Part print with two shaded views. Sizes in mm from the minimum x, y, z corner. Give positions to 0.01 mm unless a question says otherwise; leave off trailing zeros. Loops run counter-clockwise (first coordinate to the right, second up) from the corner with the lowest first, then second, coordinate; pieces in that order, holes last. Notation, with made-up numbers: M 27.5,34.5 L 59.5,34.5 A19 cw 59.5,52.5 Z; hole C -27,60.25 d8. An arc over 180 degrees is marked long. Answer in a Markdown table with one row per item.
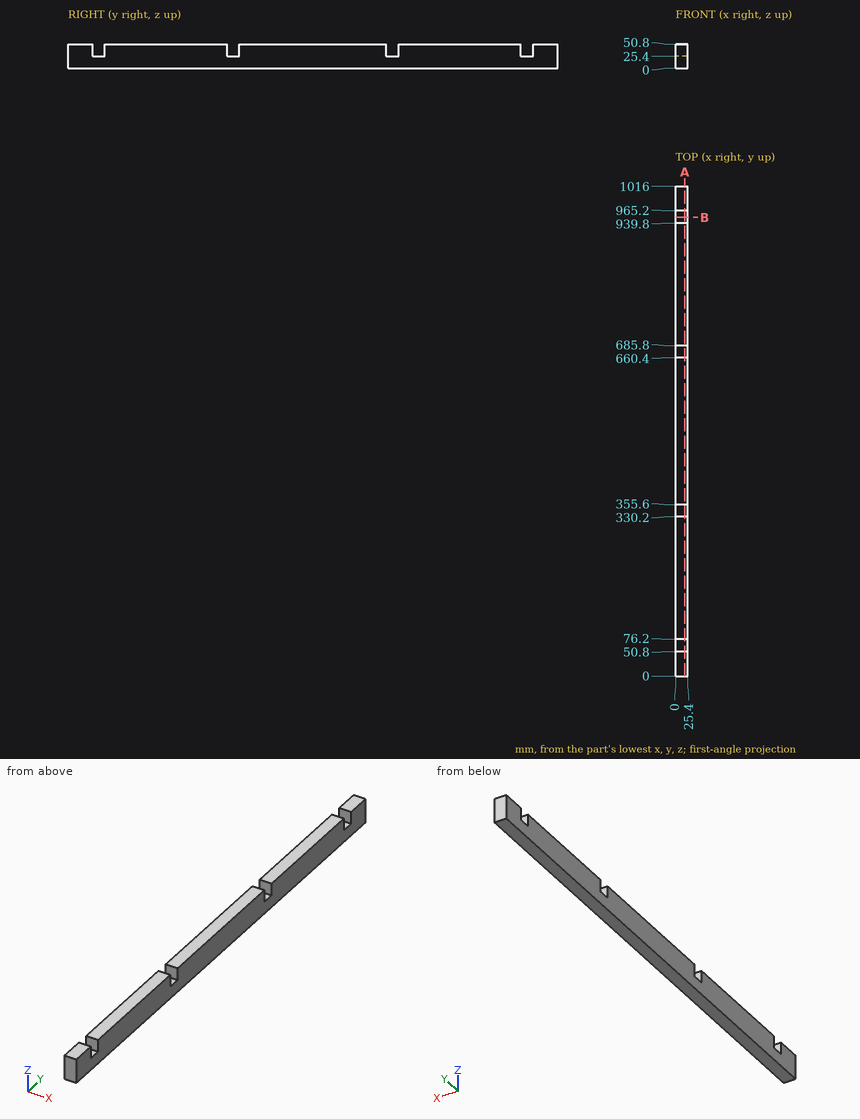
Q1. Probe probe 1 along Y at (x, z) = (24.25, 39); probe 2 along Z at (x, y) = (1, 350). List the from-to ranges inside material, lowest first.
Reported:
| item | result |
|---|---|
| probe 1 | 0 to 50.8, 76.2 to 330.2, 355.6 to 660.4, 685.8 to 939.8, 965.2 to 1016 |
| probe 2 | 0 to 25.4 |
Q2. Drop a flat-ended pin along its axis: pin 1 (7.5 mm diameter, centred on x = 11, y = 954.5, fed in from +Z). Give the stop position or say it passes through.
Reported:
| item | result |
|---|---|
| pin 1 | z = 25.4 |
Q3. Saw through at A-A (x = 19). Give the cut face in (y, z), and give its area (3 significant figures).
Reported:
| item | result |
|---|---|
| outline | M 0,0 L 1016,0 L 1016,50.8 L 965.2,50.8 L 965.2,25.4 L 939.8,25.4 L 939.8,50.8 L 685.8,50.8 L 685.8,25.4 L 660.4,25.4 L 660.4,50.8 L 355.6,50.8 L 355.6,25.4 L 330.2,25.4 L 330.2,50.8 L 76.2,50.8 L 76.2,25.4 L 50.8,25.4 L 50.8,50.8 L 0,50.8 Z |
| area | 49,000 mm² |
Q4. Saw through at B-B (y = 952). Give the cut face in (x, z), and give its area (3 significant figures).
Reported:
| item | result |
|---|---|
| outline | M 0,0 L 25.4,0 L 25.4,25.4 L 0,25.4 Z |
| area | 645 mm² |
